```python
from build123d import *

# Parameters (mm, degrees)
BOSS_EXTRUDE1_DEPTH = 20


with BuildPart() as part:
    # Sketch2 → Boss-Extrude1 (new body)
    with BuildSketch(Plane(origin=(0, 0, 0), x_dir=(0, 0, -1), z_dir=(1, 0, 0))):
        Polygon((0, 0), (80, 0), (80, 15), (60, 15), (60, 30), (80, 30), (80, 45), (55, 45), (55, 55), (80, 55), (80, 70), (60, 70), (60, 85), (80, 85), (80, 100), (0, 100), (0, 85), (20, 85), (20, 70), (0, 70), (0, 55), (25, 55), (25, 45), (0, 45), (0, 30), (20, 30), (20, 15), (0, 15), align=None)
    extrude(amount=-BOSS_EXTRUDE1_DEPTH)


solid = part.part
```
Build history of the part. All positions in model axes, mm. A direction names the side the tool comes from. Give positions to 0.01 mm unless a question says otherwise; leave off trailing zeros. Loops run counter-clockwise (first coordinate to the right, second up) from the corner with the lowest first, then second, coordinate; pieces in that order, holes last. Notation, with made-up numbers: (80.25, 69.5) - (123.25, 69.5) arc R35 cw to (123.25, 104.5) - close; hole circle Ø2 at (61, 29). An arc over 180 degrees is marked (long way). Use a Markdown table: item, result.
(1) Band-saw the part on B-B (x = -4.75). Give the cut face in (y, z), and give its area (3 significant figures).
Taken from the geometry:
| item | result |
|---|---|
| outline | (0, -80) - (15, -80) - (15, -60) - (30, -60) - (30, -80) - (45, -80) - (45, -55) - (55, -55) - (55, -80) - (70, -80) - (70, -60) - (85, -60) - (85, -80) - (100, -80) - (100, 0) - (85, 0) - (85, -20) - (70, -20) - (70, 0) - (55, 0) - (55, -25) - (45, -25) - (45, 0) - (30, 0) - (30, -20) - (15, -20) - (15, 0) - (0, 0) - close |
| area | 6,300 mm2 |
(2) Band-saw the part on C-C (y = 49.5). Give the cut face in (x, z), and give its area (3 significant figures).
Taken from the geometry:
| item | result |
|---|---|
| outline | (-20, -55) - (0, -55) - (0, -25) - (-20, -25) - close |
| area | 600 mm2 |
(3) Band-saw the part on D-D (y = 26). Give the cut face in (x, z).
Taken from the geometry:
| item | result |
|---|---|
| outline | (-20, -60) - (0, -60) - (0, -20) - (-20, -20) - close |
(4) Drop flat-ended pins along their axis: pin 1 Ø1.5 at (x, y) = (-6.5, 33.5) entering from +Z; pin 2 Ø7.5 at (x, y) = (-12, 21) entering from -Z; pin 3 Ø4.5 at (x, y) = (-5, 24.5) entering from +Z. Give the stop position or say it passes through.
Taken from the geometry:
| item | result |
|---|---|
| pin 1 | z = 0 |
| pin 2 | z = -60 |
| pin 3 | z = -20 |
(5) Band-saw the part on A-A (z = -9). Give the cut face in (x, y), and give its area (3 significant figures).
Taken from the geometry:
| item | result |
|---|---|
| outline | (-20, 0) - (0, 0) - (0, 15) - (-20, 15) - close; (-20, 30) - (0, 30) - (0, 45) - (-20, 45) - close; (-20, 55) - (0, 55) - (0, 70) - (-20, 70) - close; (-20, 85) - (0, 85) - (0, 100) - (-20, 100) - close |
| area | 1,200 mm2 |
(6) Wall check: line 1 along Y through (x, z) = (-10, -18.5); line 2 along Y through (x, z) = (-1.25, -56); line 3 along Z through (x, y) = (-13.75, 54). Give the ranges that are in metal, low to high.
Taken from the geometry:
| item | result |
|---|---|
| line 1 | 0 to 15, 30 to 45, 55 to 70, 85 to 100 |
| line 2 | 0 to 45, 55 to 100 |
| line 3 | -55 to -25 |
(7) Pull direction Y, two halves, no side cores. Call faces 4 (the face through (-20, 51, -39)), 5 (the face through (-10, 70, -10)), 6 (the face through (-10, 70, -70)), 7 (the face through (-10, 0, -39)): +Y half, -Y half, draft (parallel to the pull), parting line (faces both ways), or undercut.
Taken from the geometry:
| item | result |
|---|---|
| face 4 | draft |
| face 5 | undercut |
| face 6 | undercut |
| face 7 | -Y half |
(8) Which spindle directions (+Z, -Z, +X, -X, +Y, -Y) get a long thin tool onto all of the face, cutting with end or side? Do faces 1 (the face through (-10, 23, -20)), 2 (the face through (-10, 15, -70)), 3 (the face through (-10, 62, -80)). Say none if no direction does.
Taken from the geometry:
| item | result |
|---|---|
| face 1 | +Z, +X, -X |
| face 2 | -Z, +X, -X |
| face 3 | -Z, +X, -X, +Y, -Y |
